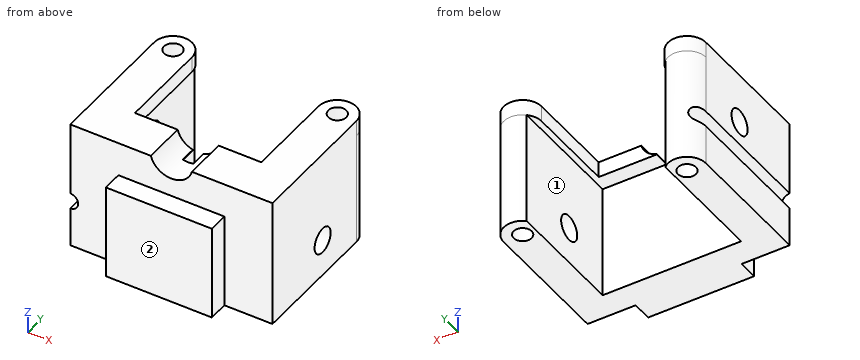
Autodesk Inventor part; units mm, degrees
ref_plane "YZ Plane" through (0, 0, 0) normal (1, 0, 0) x (0, 1, 0)
ref_plane "XZ Plane" through (0, 0, 0) normal (0, 1, 0) x (-1, 0, 0)
ref_plane "XY Plane" through (0, 0, 0) normal (0, 0, 1) x (1, 0, 0)
sketch "Sketch1" plane through (0, 0, 0) normal (0, 0, 1) x (1, 0, 0)
  line L0 (-13.075, 0) -> (13.075, 0)
  line L1 (13.075, 0) -> (13.075, 22.6856)
  line L2 (-13.075, 22.6856) -> (-13.075, 0)
  line L3 (-19.075, -5) -> (11.925, -5)
  line L4 (19.075, -5) -> (19.075, 20.0588)
  line L5 (-19.075, 20.0588) -> (-19.075, -5)
  circle A0 centre (-15.5, 20.0588) radius 1.5
  circle A1 centre (15.5, 20.0588) radius 1.5
  arc A2 (19.075, 20.0588) -> (13.075, 22.6856) centre (15.5, 20.0588) ccw
  arc A3 (-13.075, 22.6856) -> (-19.075, 20.0588) centre (-15.5, 20.0588) ccw
  line L6 (11.925, -5) -> (19.075, -5)
  point P0 (0, 0)
  dimension "d8" = 5
  dimension "d10" = 6
  dimension "d12" = 31
  dimension "d14" = 3
  dimension "d15" = 3
  dimension "d17" = 26.15
  dimension "d18" = 13.075
  dimension "d19" = 15.5
extrude "Extrusion1" add sketch "Sketch1" along normal blind 20.5 contours L0 L1 A2 L4 L6 L3 L5 A3 L2 | A0 | A1
sketch "Sketch4" plane through (0, 0, 20.5) normal (0, 0, 1) x (1, 0, 0)
  arc A0 (-11.925, 20.0588) -> (-19.075, 20.0588) centre (-15.5, 20.0588) ccw
  arc A1 (19.075, 20.0588) -> (11.925, 20.0588) centre (15.5, 20.0588) ccw
  arc A2 (19.075, 20.0588) -> (13.075, 22.6856) centre (15.5, 20.0588) ccw
  arc A3 (-13.075, 22.6856) -> (-19.075, 20.0588) centre (-15.5, 20.0588) ccw
  line L0 (-19.075, -5) -> (19.075, -5)
  line L1 (19.075, -5) -> (19.075, 20.0588)
  arc A4 (19.075, 20.0588) -> (13.075, 22.6856) centre (15.5, 20.0588) ccw
  line L2 (13.075, 22.6856) -> (13.075, 0)
  line L3 (13.075, 0) -> (-13.075, 0)
  line L4 (-13.075, 0) -> (-13.075, 22.6856)
  arc A5 (-13.075, 22.6856) -> (-19.075, 20.0588) centre (-15.5, 20.0588) ccw
  line L5 (-19.075, 20.0588) -> (-19.075, -5)
  line L6 (-11.925, 20.0588) -> (-11.925, 3)
  line L7 (-11.925, 3) -> (11.925, 3)
  line L8 (11.925, 3) -> (11.925, 20.0588)
  point P0 (0, 0)
  point P1 (13.075, 22.6856)
  point P2 (13.075, 22.6856)
  dimension "d37" = 3
extrude "Extrusion3" add sketch "Sketch4" along normal blind 3
sketch "Sketch5" plane through (0, 0, 23.5) normal (0, 0, 1) x (1, 0, 0)
  arc A0 (-13.075, 22.6856) -> (-19.075, 20.0588) centre (-15.5, 20.0588) ccw
  arc A1 (19.075, 20.0588) -> (13.075, 22.6856) centre (15.5, 20.0588) ccw
  point P0 (0, 0)
hole "Hole2" at (-15.5, 20.0588, 23.5) at (15.5, 20.0588, 23.5) direction (0, 0, -1) diameter 3.4 end through all
sketch "Sketch8" plane through (-13.075, 0, 0) normal (0, 1, 0) x (1, 0, 0)
  circle A0 centre (13.075, -24.5) radius 4
  line L0 (25, -23.5) -> (1.15, -23.5)
  point P0 (13.075, 0)
  dimension "d62" = 8
  dimension "d63" = 1
extrude "Extrusion5" cut sketch "Sketch8" against normal through all both and the other way through all
sketch "Sketch9" plane through (-13.075, 0, 0) normal (0, 1, 0) x (1, 0, 0)
  line L0 (12.075, -28.8924) -> (14.075, -28.8924)
  line L1 (14.075, -28.8924) -> (14.075, -18.1034)
  line L2 (14.075, -18.1034) -> (12.075, -18.1034)
  line L3 (12.075, -18.1034) -> (12.075, -28.8924)
  line L4 (12.075, -28.8924) -> (14.075, -18.1034) construction
  line L5 (14.075, -28.8924) -> (12.075, -18.1034) construction
  point P0 (13.075, 0)
  point P1 (13.075, -23.4979)
  dimension "d66" = 2
extrude "Extrusion6" cut sketch "Sketch9" along normal blind 10
sketch "Sketch10" plane through (19.075, -5, 0) normal (1, 0, 0) x (0, 0, -1)
  circle A0 centre (-6, 14.9996) radius 2
  line L0 (0, 0) -> (-23.5, 0)
  line L1 (0, 0) -> (0, 25.0588)
  line L2 (0, 27.6856) -> (-20.5, 27.6856)
  point P0 (0, 5)
  dimension "d70" = 6
  dimension "d71" = 4
  dimension "d88" = 12.686
hole "Hole4" at (19.075, 9.9996, 6) direction (-1, 0, 0) diameter 4.8 depth 6
sketch "Sketch11" plane through (-19.075, -5, 0) normal (-1, 0, 0) x (0, 0, 1)
  circle A0 centre (14, 14.9996) radius 3.2686
  line L0 (0, 0) -> (23.5, 0)
  circle A1 centre (6, 14.9996) radius 2.4
  line L1 (0, 27.6856) -> (20.5, 27.6856)
  point P0 (0, 5)
  point P1 (10.9595, 8.3093)
  dimension "d80" = 8
  dimension "d89" = 12.686
hole "Hole5" at (-19.075, 9.9996, 14) direction (1, 0, 0) diameter 4.8 depth 6
sketch "Sketch12" plane through (-19.075, -5, 0) normal (0, -1, 0) x (1, 0, 0)
  line L0 (38.15, 0) -> (38.15, 23.5)
  circle A0 centre (0, 8) radius 1.5
  line L1 (0, 0) -> (0, 23.5)
  line L2 (0, 0) -> (38.15, 0)
  point P0 (19.075, 0)
  dimension "d93" = 3
  dimension "d94" = 8
extrude "Extrusion7" cut sketch "Sketch12" against normal through all
sketch "Sketch13" plane through (0, 0, 0) normal (0, 0, -1) x (-1, 0, 0)
  circle A0 centre (15.5, 20.0588) radius 1.7
  circle A1 centre (-15.5, 20.0588) radius 1.7
  line L0 (19.075, 20.0588) -> (19.075, -5)
  arc A2 (19.075, 20.0588) -> (13.075, 22.6856) centre (15.5, 20.0588) ccw
  line L1 (13.075, 0) -> (13.075, 22.6856)
  line L2 (-13.075, 0) -> (13.075, 0)
  line L3 (-13.075, 22.6856) -> (-13.075, 0)
  arc A3 (-13.075, 22.6856) -> (-19.075, 20.0588) centre (-15.5, 20.0588) ccw
  line L4 (-19.075, -5) -> (-19.075, 20.0588)
  line L5 (19.075, -5) -> (-19.075, -5)
  line L6 (-4.8329, -8.7412) -> (5.1671, -8.7412)
  line L7 (-10, -1.2588) -> (10, -1.2588)
  line L8 (10, -1.2588) -> (10, -8.7412)
  line L9 (10, -8.7412) -> (-10, -8.7412)
  line L10 (-10, -8.7412) -> (-10, -1.2588)
  line L11 (19.075, -5) -> (-19.075, -5)
  line L12 (-10, -1.2588) -> (10, -8.7412) construction
  line L13 (10, -1.2588) -> (-10, -8.7412) construction
  point P0 (0, 0)
  point P1 (0, -5)
  point P2 (-10, -5)
  point P3 (10, -5)
  dimension "d95" = 20
extrude "Extrusion8" add sketch "Sketch13" against normal blind 17 contours L8 L9 L6 L10 L5
move faces "Move1" translate (0, 0, -1) faces at (-17.075, 5.0196, 0)
properties part number "SolenoidBracket"
Could you check a few things on this model? Use its own coordinates, in mm. Face numbers are marked on the shaded views. A direction names the side the tool comes from. Coordinates: 2 decimals unless noted, no trailing zeros. Loops run counter-clockwise (first coordinate to the right, second up) from the corner with the lowest first, then second, coordinate; pieces in that order, holes last. Notation, with made-up numbers: (-4.5, 32) -> (47.5, 32) arc R25 ccw to (47.5, 44) -> close; hole circle Ø9 at (-22, -31.5). An arc over 180 degrees is marked (long way). Answer in a Markdown table with one row per item.
(1) For the marked faces 1 and 2, which set-ups out of +Z, -Z, +X, -X, +Y, -Y let a thin tool reach every point of the face, with its end or its side?
Results found:
| item | result |
|---|---|
| face 1 | -Z, +Y |
| face 2 | +Z, -Z, +X, -X, -Y |
(2) If I drill on probe 1 along X at (y, z) = (3.5, 21.25) (3 decimals); probe 2 along X at (y, z) = (1, 14) (3 decimals); probe 3 along X at (y, z) = (18.5, 12) (3 decimals), over which ranges is the centre line in solid material (lowest first)?
Results found:
| item | result |
|---|---|
| probe 1 | x = -19.075 to -11.925, 11.925 to 19.075 |
| probe 2 | x = -19.075 to -13.075, 13.075 to 19.075 |
| probe 3 | x = -19.075 to -16.178, -14.822 to -13.075, 13.075 to 14.822, 16.178 to 19.075 |
(3) Imagine slicing it at C-C (z = 10). List the corners of the cut face in (x, y) for me (3 decimals).
Results found:
| item | result |
|---|---|
| outline | (-19.075, -5) -> (-10, -5) -> (-10, -8.741) -> (10, -8.741) -> (10, -5) -> (19.075, -5) -> (19.075, 20.059) arc R3.575 ccw to (13.075, 22.686) -> (13.075, 0) -> (-13.075, 0) -> (-13.075, 22.686) arc R3.575 ccw to (-19.075, 20.059) -> close; hole circle Ø3.4 at (-15.5, 20.059); hole circle Ø3.4 at (15.5, 20.059) |
(4) Imagine slicing it at D-D (x = -15.5). List the corners of the cut face in (y, z) for me, plus the area to 3 significant figures.
Results found:
| item | result |
|---|---|
| outline | (-5, -1) -> (18.36, -1) -> (18.36, 23.5) -> (-5, 23.5) -> close; (21.76, -1) -> (23.63, -1) -> (23.63, 23.5) -> (21.76, 23.5) -> close; hole circle Ø4.8 at (10, 14) |
| area | 600 mm^2 |
(5) Imagine slicing it at B-B (z = 5.25). List the corners of the cut face in (x, y) for me (3 decimals), plus the area to 3 significant figures.
Results found:
| item | result |
|---|---|
| outline | (-19.075, -5) -> (-10, -5) -> (-10, -8.741) -> (10, -8.741) -> (10, -5) -> (19.075, -5) -> (19.075, 7.72) -> (13.075, 7.72) -> (13.075, 0) -> (-13.075, 0) -> (-13.075, 22.686) arc R3.575 ccw to (-19.075, 20.059) -> close; (13.075, 12.279) -> (19.075, 12.279) -> (19.075, 20.059) arc R3.575 ccw to (13.075, 22.686) -> close; hole circle Ø3.4 at (-15.5, 20.059); hole circle Ø3.4 at (15.5, 20.059) |
| area | 497 mm^2 |
(6) Imagine slicing it at A-A (y = 5.5). List the corners of the cut face in (x, z) for me (3 decimals), plus the area to 3 significant figures.
Results found:
| item | result |
|---|---|
| outline | (-19.075, -1) -> (-13.075, -1) -> (-13.075, 20.5) -> (-11.925, 20.5) -> (-11.925, 23.5) -> (-19.075, 23.5) -> (-19.075, 9.5) arc R1.5 cw to (-19.075, 6.5) -> close; (11.925, 20.5) -> (13.075, 20.5) -> (13.075, -1) -> (19.075, -1) -> (19.075, 23.5) -> (11.925, 23.5) -> close |
| area | 297 mm^2 |
(7) Will these pins go through, and if not, where does the flat tip stop? pin 1 Ø3 at (x, z) = (3.5, 8) entering from +Y; pin 2 Ø5 at (x, z) = (-6, 18.5) entering from +Y; pin 3 Ø6 at (x, z) = (-11, 12) entering from +Y.
Results found:
| item | result |
|---|---|
| pin 1 | stops at y = 0 |
| pin 2 | stops at y = 3 |
| pin 3 | stops at y = 23.3 |
